Answer from the drawing. Dimensions are ordinates in mm from the lowest x, y and z of the part. A direction names the side the tool comes from. Give positions to 0.01 mm unless a question says otherwise; leave off trailing zeros. Order: outer loops, then holes, each group sorted by start corner. A loop starts at its lowest first (then second) coordinate and runs counter-clockwise, first axis right, second up.
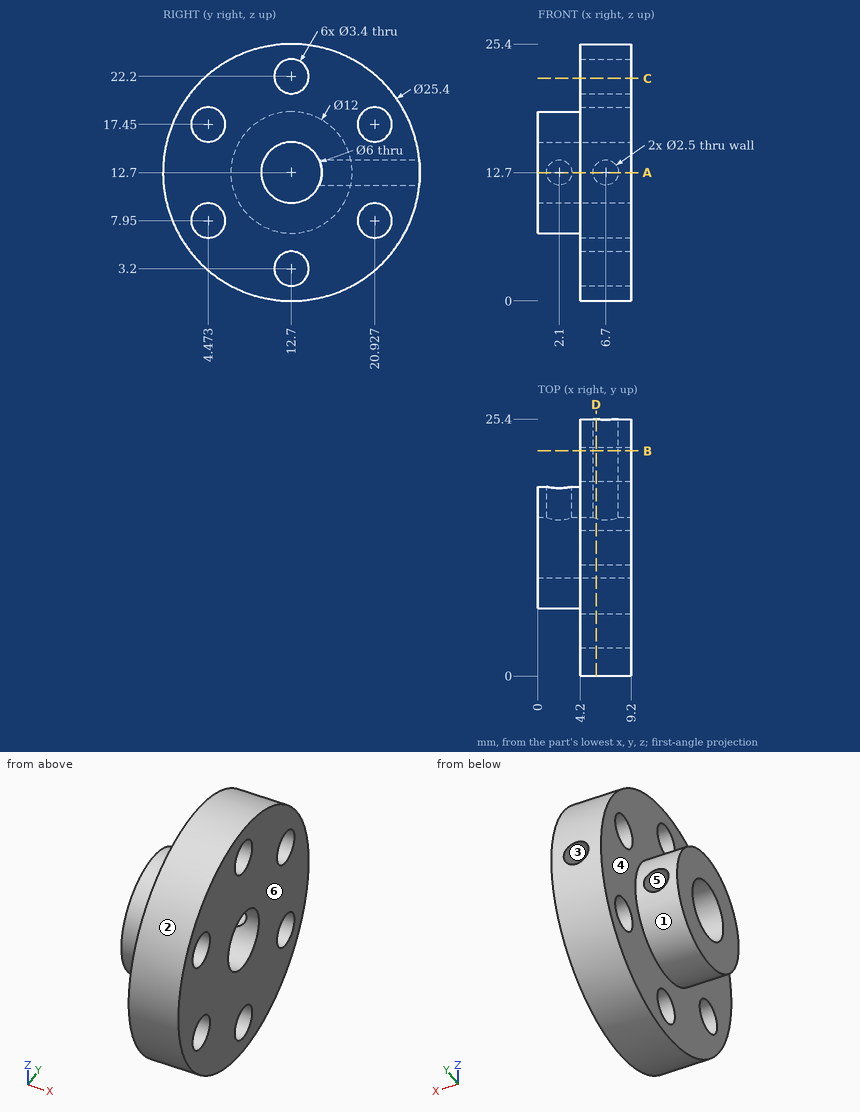
1) Consider L1, parallel to Y at x = 7.95, z = 7.95; L2, parallel to Y at x = 6, z = 18.75 (1 decimal); L3, parallel to X at y = 22.5, z = 12.7. Determine where each line is inside the solid, lowest interval first.
Final values:
L1: y = 0.92 to 2.77, 6.17 to 19.23, 22.63 to 24.48
L2: y = 1.5 to 3.4, 5.6 to 19.8, 22 to 23.9
L3: x = 4.2 to 5.45, 7.95 to 9.2
2) A tool of negligible diameter and unlimited length cuts with its end or side. For the marked faces 1, 2 and 3, from which of +Z, -Z, +X, -X, +Y, -Y can it reach the whole face along a straight path? Write none if from no direction.
Final values:
face 1: -X
face 2: +X, -X
face 3: +Y
3) The part is cut by section D-D on x = 5.75. Determine the outline of the cut face in (y, z).
Final values:
outline: (15.59, 11.89) arc R3 cw (long way) to (15.59, 13.51) - (25.37, 13.51) arc R12.7 ccw (long way) to (25.37, 11.89) - close; hole circle Ø3.4 at (4.47, 7.95); hole circle Ø3.4 at (4.47, 17.45); hole circle Ø3.4 at (12.7, 3.2); hole circle Ø3.4 at (12.7, 22.2); hole circle Ø3.4 at (20.93, 7.95); hole circle Ø3.4 at (20.93, 17.45)
4) Given pin 1 (1.5 mm diameter, centred on y = 3, z = 14.5, fed in from -X); pin 2 (2 mm diameter, centred on y = 12.7, z = 3.2, fed in from -X); pin 3 (1.5 mm diameter, centred on x = 2.1, z = 12.7, fed in from +Y) (1 decimal); pin 4 (4 mm diameter, centred on x = 3.5, z = 19.5, fed in from -Y) (1 decimal), each flat-ended and moving along its own axis, determine where each tip first touches the part or whether it passes through.
Final values:
pin 1: stops at x = 4.2
pin 2: passes through
pin 3: stops at y = 9.8
pin 4: stops at y = 1
5) The part is cut by section B-B on y = 22.25. Determine the outline of the cut face in (x, z).
Final values:
outline: (4.2, 4.33) - (9.2, 4.33) - (9.2, 6.88) - (4.2, 6.88) - close; (4.2, 9.02) - (9.2, 9.02) - (9.2, 16.38) - (4.2, 16.38) - close; (4.2, 18.52) - (9.2, 18.52) - (9.2, 21.07) - (4.2, 21.07) - close; hole circle Ø2.5 at (6.7, 12.7)
6) For a pull along X with two mould halves and no side action, classify the marked faces 4, 5 and 6 as released by +X, released by -X, zero draft, split by the parting line, or undercut.
Final values:
face 4: released by -X
face 5: undercut
face 6: released by +X
7) The part is cut by section C-C on z = 22. Determine the outline of the cut face in (x, y).
Final values:
outline: (4.2, 4.05) - (9.2, 4.05) - (9.2, 11.01) - (4.2, 11.01) - close; (4.2, 14.39) - (9.2, 14.39) - (9.2, 21.35) - (4.2, 21.35) - close
8) The part is cut by section A-A on z = 12.7. Determine the outline of the cut face in (x, y).
Final values:
outline: (0, 6.7) - (4.2, 6.7) - (4.2, 0) - (9.2, 0) - (9.2, 9.7) - (0, 9.7) - close; (0, 15.7) - (0.85, 15.7) - (0.85, 18.7) - (0, 18.7) - close; (3.35, 15.7) - (5.45, 15.7) - (5.45, 25.4) - (4.2, 25.4) - (4.2, 18.7) - (3.35, 18.7) - close; (7.95, 15.7) - (9.2, 15.7) - (9.2, 25.4) - (7.95, 25.4) - close
